Geometry check sheet. Reference: the model listing, model coordinates, mm. A direction names the side the tool comes from. Coordinates: 2 decimals unless noted, no trailing zeros. Write each loop counter-clockwise with the first axis right and the second up, starting at its lowest first coordinate (ties: lowest second). Pieces come first, ordered by that corner, then holes. Notation, with made-up numbers: (76, 87.25) -> (99, 87.25) arc R10 ccw to (99, 99.25) -> close; hole circle Ø4 at (33.25, 45.25). An arc over 180 degrees is marked (long way). Answer in a Markdown table with one row per item. Add a question column.
1. Scan lines: L1, parallel to X at y = 7.5, z = 3.75; L2, parallel to X at y = -4.5, z = 2.25; L3, parallel to Z at x = 5.5, y = -12.5. Record each from-to range of solid material in increasing order. Write a range as from..to.
2. Mould release check, pull along Y, two halves, no side actions. Record for faces 1 (the flat face through (0, 0, 16)), 2 (the cylindrical face through (0.68, -13.715, 1.301)), 3 (the cylindrical face through (6.445, 5.979, 3.014)): pulls with the +Y half, pulls with the -Y half, needs draft (parallel to the pull), parting line crosses it, or undercut.
3. Set-up check for faces 4 (the flat face through (-3, -3, 0)), 5 (the cylindrical face through (-13.715, -13.699, 3.014)): record each of +Z, -Z, +X, -X, +Y, -Y from which the full face is reachable in a straight line by a thin tool's end or side.
4. Depth check by flat-ended pin: P1, Ø1.5, axis at y = -5.5, z = 11, coming from the -X side; P2, Ø2, axis at y = -2.5, z = 3, coming from the +X side; P3, Ø12, axis at x = 0.5, y = 7.5, coming from the +Z side; P4, Ø3, axis at x = -9.5, z = 2, coming from the +Y side. Enter the tip coordinate at first touch or a pass-through.
5. Cross-section at A-A on z = 2.75. Record the cut outline in (x, y), and give its area (3 significant figures).
```python
from build123d import *

# Parameters (mm, degrees)
SKETCH_1_W          = 30
SKETCH_1_H          = 30
EXTRUDE_1_DEPTH     = 4
CUT_EXTRUDE_1_DEPTH = 22.587033145
FILLET_1_R          = 2
SHELL_1_T           = -1
SKETCH_2_R          = 3.4
EXTRUDE_2_DEPTH     = 15


with BuildPart() as part:
    # 草图1 → 凸台-拉伸1 (new body)
    with BuildSketch(Plane.XY):
        Rectangle(SKETCH_1_W, SKETCH_1_H)
    extrude(amount=EXTRUDE_1_DEPTH)

    # 草图4 → 切除-拉伸1 (cut, through all)
    with BuildSketch(Plane.XY.offset(4)):
        with BuildLine():
            Line((-15, 15), (15, 15))
            Line((15, 15), (15, -15))
            ThreePointArc((15, -15), (6.213203436, 6.213203436), (-15, 15))
        make_face()
    extrude(amount=-CUT_EXTRUDE_1_DEPTH, mode=Mode.SUBTRACT)

    # 圆角1
    fillet_1_edges = [part.edges().sort_by_distance(p)[0] for p in [
        (6.213203436, 6.213203436, 0),
        (0, -15, 0),
        (-15, 0, 0),
        (-15, -15, 2),
    ]]
    fillet(fillet_1_edges, radius=FILLET_1_R)

    # 抽壳1
    shell_1_openings = [part.faces().sort_by_distance(p)[0] for p in [
        (-2.252666732, -2.252666732, 4),
    ]]
    offset(amount=SHELL_1_T, openings=shell_1_openings)

    # 草图2 → 凸台-拉伸2 (add)
    with BuildSketch(Plane.XY.offset(1)):
        Circle(SKETCH_2_R)
    extrude(amount=EXTRUDE_2_DEPTH)


solid = part.part
```
Results found:
| question | item | result |
|---|---|---|
| 1 | L1 | x = -15..-14, 3.3..4.84 |
| 1 | L2 | x = -15..-14, 12.03..13.1 |
| 1 | L3 | z = 0..1 |
| 2 | face 1 | needs draft |
| 2 | face 2 | undercut |
| 2 | face 3 | pulls with the +Y half |
| 3 | face 4 | -Z, +X, -X, +Y, -Y |
| 3 | face 5 | +Z |
| 4 | P1 | passes through |
| 4 | P2 | stops at x = 12.71 |
| 4 | P3 | stops at z = 16 |
| 4 | P4 | stops at y = 14.73 |
| 5 | outline | (-15, -13) arc R2 ccw to (-13, -15) -> (15, -15) arc R30 ccw to (-15, 15) -> close; circle Ø6.8 at (0, 0); hole (-14, -13) arc R1 ccw to (-13, -14) -> (13.98, -14) arc R29 ccw to (-14, 13.98) -> close |
| 5 | area | 139 mm^2 |
